Verification items for this drawing (mm, ordinates from the low corner). Give positions to 0.01 mm unless a question says otherwise; leave off trailing zeros. Write each loop counter-clockwise with the first axis right and the second up, starting at its lowest first coordinate (ties: lowest second). Pieces come first, ordered by that corner, then holes. Notation, with made-up numbers: (77, 84) -> (98, 84) arc R21 ccw to (98, 92) -> close; hole circle Ø8 at (86, -15). An arc over 180 degrees is marked (long way). One line per item, written item: value.
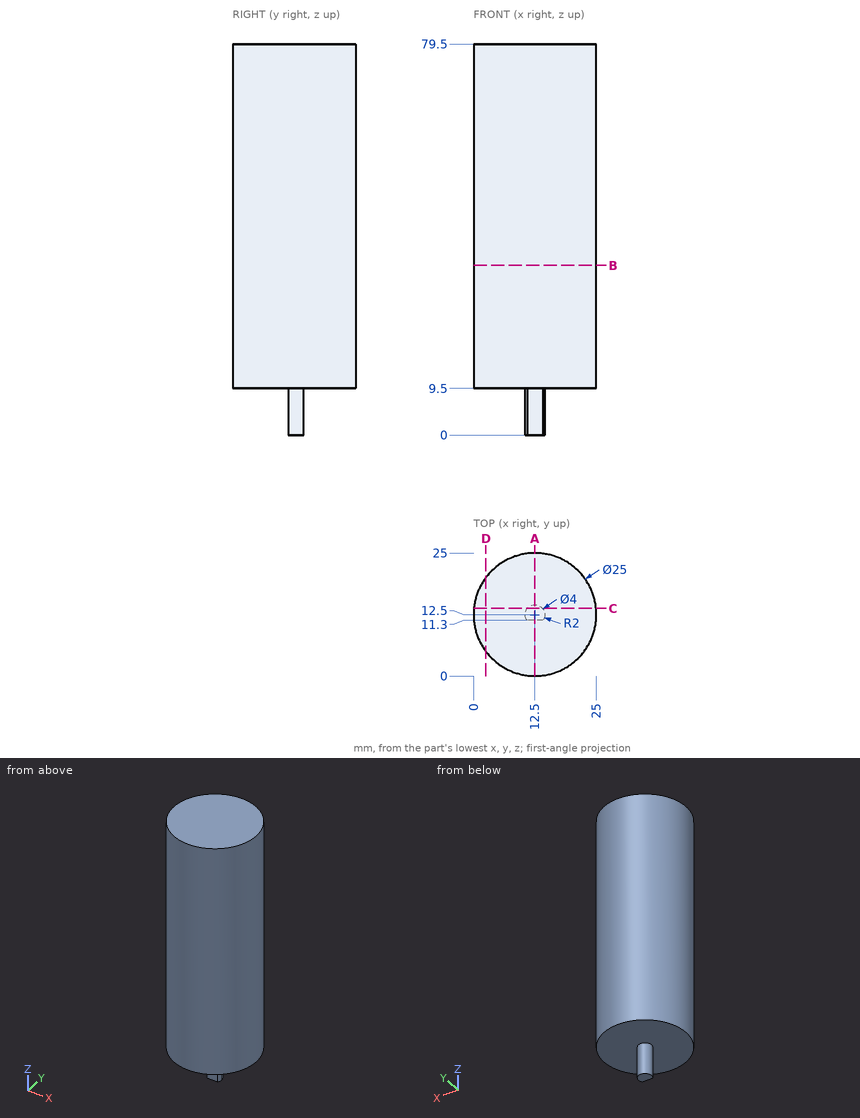
1) Sectioned sample at A-A on x = 12.5. Record the cut outline in (y, z), plus the area to 3 significant figures.
Verdict:
outline: (0, 9.5) -> (11.3, 9.5) -> (11.3, 0) -> (14.5, 0) -> (14.5, 9.5) -> (25, 9.5) -> (25, 79.5) -> (0, 79.5) -> close
area: 1,780 mm^2
2) Sectioned sample at B-B on z = 34.5. Record the cut outline in (x, y), plus the area to 3 significant figures.
Verdict:
outline: circle Ø25 at (12.5, 12.5)
area: 491 mm^2
3) Sectioned sample at D-D on x = 2.5. Record the cut outline in (y, z), plus the area to 3 significant figures.
Verdict:
outline: (5, 9.5) -> (20, 9.5) -> (20, 79.5) -> (5, 79.5) -> close
area: 1,050 mm^2
4) Sectioned sample at C-C on y = 13.75. Record the cut outline in (x, z), plus the area to 3 significant figures.
Verdict:
outline: (0.06, 9.5) -> (10.94, 9.5) -> (10.94, 0) -> (14.06, 0) -> (14.06, 9.5) -> (24.94, 9.5) -> (24.94, 79.5) -> (0.06, 79.5) -> close
area: 1,770 mm^2
5) Scan lines: probe 1 along Z at (x, y) = (22.75, 17); probe 2 along Y at (x, z) = (13, 36); probe 3 along X at (y, z) = (20.5, 34). Record each from-to range of solid material in increasing order.
Verdict:
probe 1: 9.5 to 79.5
probe 2: 0.01 to 24.99
probe 3: 2.9 to 22.1
6) Depth check by flat-ended pin: pin 1 Ø1 at (y, z) = (13.5, 59) entering from -X; pin 2 Ø8 at (x, z) = (6.5, 10) entering from -Y; pin 3 Ø5 at (x, y) = (6.5, 6) entering from -Z. Enter the tip coordinate at first touch or a pass-through.
Verdict:
pin 1: x = 0.01
pin 2: y = 0.16
pin 3: z = 9.5
